```python
from build123d import *

# Parameters (mm, degrees)
F0_W      = 150
F0_H      = 98.5
F1_DEPTH  = 5
F3_W      = 70.65
F3_H      = 77.55
F3_W_2    = 68.65
F3_H_2    = 75.55
F4_DEPTH  = 1
F5_R      = 4
F5_R_2    = 2
F6_DEPTH  = 3
F7_R      = 1.5
F8_DEPTH  = 12.5
F9_R      = 2.75
F10_DEPTH = 2.5
F11_W     = 3
F11_H     = 10
F12_DEPTH = 25
F14_DEPTH = 5
F15_R     = 4
F16_DEPTH = 25
F13_W     = 1
F13_H     = 6
F17_DEPTH = 25
F18_W     = 9.35
F18_H     = 6
F19_DEPTH = 2
F20_W     = 10
F20_H     = 3
F21_DEPTH = 5
F23_DEPTH = 200


with BuildPart() as f1:
    # F0 (on Top) → F1 (new body)
    with BuildSketch(Plane.XY):
        Rectangle(F0_W, F0_H)
    extrude(amount=F1_DEPTH)

    # F3 (on face) → F4 (join)
    with BuildSketch(Plane.XY.offset(5)):
        Polygon((-66.5, -42.5), (-66.5, 42.5), (-67.5, 43.5), (-67.5, -43.5), align=None)
        Polygon((-12.5, 43.5), (-13.5, 42.5), (-13.5, -42.5), (-12.5, -43.5), align=None)
        with Locations((32.175, -0.275)):
            Rectangle(F3_W, F3_H)
        with Locations((32.175, -0.275)):
            Rectangle(F3_W_2, F3_H_2, mode=Mode.SUBTRACT)
    extrude(amount=F4_DEPTH)

    # F5 (on face) → F6 (join)
    with BuildSketch(Plane.XY.offset(5)):
        with Locations((9, 27.5)):
            Circle(F5_R)
        with Locations((9, 27.5)):
            Circle(F5_R_2, mode=Mode.SUBTRACT)
        with Locations((55.5, 27.5)):
            Circle(F5_R)
        with Locations((55.5, 27.5)):
            Circle(F5_R_2, mode=Mode.SUBTRACT)
        with Locations((55.5, -23)):
            Circle(F5_R)
        with Locations((55.5, -23)):
            Circle(F5_R_2, mode=Mode.SUBTRACT)
        with Locations((9, -23)):
            Circle(F5_R)
        with Locations((9, -23)):
            Circle(F5_R_2, mode=Mode.SUBTRACT)
    extrude(amount=F6_DEPTH)

    # F7 (on face) → F8 (cut, symmetric)
    with BuildSketch(Plane.XY.offset(5)):
        with Locations((9, 27.5)):
            Circle(F7_R)
        with Locations((55.5, 27.5)):
            Circle(F7_R)
        with Locations((9, -23)):
            Circle(F7_R)
        with Locations((55.5, -23)):
            Circle(F7_R)
        with Locations((-58, 33.5)):
            Circle(F7_R)
        with Locations((-22, 33.5)):
            Circle(F7_R)
        with Locations((-58, -33.5)):
            Circle(F7_R)
        with Locations((-22, -33.5)):
            Circle(F7_R)
        with Locations((-60, -44.25)):
            Circle(F7_R)
        with Locations((60, -44.25)):
            Circle(F7_R)
        with Locations((60, 44.25)):
            Circle(F7_R)
        with Locations((-60, 44.25)):
            Circle(F7_R)
    extrude(amount=F8_DEPTH, both=True, mode=Mode.SUBTRACT)

    # F9 (on face) → F10 (cut)
    with BuildSketch(Plane(origin=(0, 0, 0), x_dir=(1, 0, 0), z_dir=(0, 0, -1))):
        with Locations((9, 23)):
            Circle(F9_R)
        with Locations((55.5, 23)):
            Circle(F9_R)
        with Locations((9, -27.5)):
            Circle(F9_R)
        with Locations((55.5, -27.5)):
            Circle(F9_R)
        with Locations((-22, -33.5)):
            Circle(F9_R)
        with Locations((-58, -33.5)):
            Circle(F9_R)
        with Locations((-22, 33.5)):
            Circle(F9_R)
        with Locations((-58, 33.5)):
            Circle(F9_R)
        with Locations((-60, -44.25)):
            Circle(F9_R)
        with Locations((60, -44.25)):
            Circle(F9_R)
        with Locations((-60, 44.25)):
            Circle(F9_R)
        with Locations((60, 44.25)):
            Circle(F9_R)
    extrude(amount=-F10_DEPTH, mode=Mode.SUBTRACT)

    # F11 (on face) → F12 (cut)
    with BuildSketch(Plane.XY.offset(5)):
        with Locations((-71.5, 30)):
            Rectangle(F11_W, F11_H)
        with Locations((-71.5, 0)):
            Rectangle(F11_W, F11_H)
        with Locations((-71.5, -30)):
            Rectangle(F11_W, F11_H)
        with Locations((71.5, -30)):
            Rectangle(F11_W, F11_H)
        with Locations((71.5, 30)):
            Rectangle(F11_W, F11_H)
        with Locations((71.5, 0)):
            Rectangle(F11_W, F11_H)
    extrude(amount=-F12_DEPTH, mode=Mode.SUBTRACT)

    # F13 (on face) → F14 (join)
    with BuildSketch(Plane.XY.offset(5)):
        Polygon((-7.825, 29.25), (-12.5, 29.25), (-12.5, 27.25), (-11.5, 27.25), (-11.5, 21.25), (-12.5, 21.25), (-12.5, 19.25), (-7.825, 19.25), align=None)
        Polygon((-3.15, 29.25), (-7.825, 29.25), (-7.825, 19.25), (-3.15, 19.25), (-3.15, 21.25), (-4.15, 21.25), (-4.15, 27.25), (-3.15, 27.25), align=None)
    extrude(amount=F14_DEPTH)

    # F15 (on face) → F16 (cut)
    with BuildSketch(Plane.XZ.offset(-19.25)):
        with Locations((-7.825, 10)):
            Circle(F15_R)
    extrude(amount=-F16_DEPTH, mode=Mode.SUBTRACT)

    # F13 (on face) → F17 (cut)
    with BuildSketch(Plane.XY.offset(5)):
        with Locations((-12, 24.25)):
            Rectangle(F13_W, F13_H)
        with Locations((-3.65, 24.25)):
            Rectangle(F13_W, F13_H)
    extrude(amount=-F17_DEPTH, mode=Mode.SUBTRACT)

    # F18 (on face) → F19 (cut)
    with BuildSketch(Plane(origin=(0, 0, 0), x_dir=(1, 0, 0), z_dir=(0, 0, -1))):
        with Locations((-7.825, -24.25)):
            Rectangle(F18_W, F18_H)
    extrude(amount=-F19_DEPTH, mode=Mode.SUBTRACT)

    # F20 (on face) → F21 (join)
    with BuildSketch(Plane(origin=(0, 49.25, 0), x_dir=(-1, 0, 0), z_dir=(0, 1, 0))):
        with Locations((-62.5, 3.5)):
            Rectangle(F20_W, F20_H)
        with Locations((-27.5, 3.5)):
            Rectangle(F20_W, F20_H)
        with Locations((27.5, 3.5)):
            Rectangle(F20_W, F20_H)
        with Locations((62.5, 3.5)):
            Rectangle(F20_W, F20_H)
    extrude(amount=F21_DEPTH)

    # F22 (on face) → F23 (cut)
    with BuildSketch(Plane(origin=(-67.5, 0, 0), x_dir=(0, -1, 0), z_dir=(-1, 0, 0))):
        Polygon((-54.25, 5), (-54.25, 3.5), (-51.75, 5), align=None)
    extrude(amount=-F23_DEPTH, mode=Mode.SUBTRACT)


solid = f1.part
```
Check sheet for the modelled part. Datum: model origin and axes. Units: mm. A direction names the side the tool comes from. Round coordinates to 2 decimals unless told otherwise and drop trailing zeros. Loops run counter-clockwise (first coordinate to the right, second up) from the corner with the lowest first, then second, coordinate; pieces in that order, holes last. Notation, with made-up numbers: (-33.75, -25) -> (3.25, -25) arc R19 ccw to (3.25, -17) -> close; hole circle Ø3 at (64, -39). An arc over 180 degrees is marked (long way). Write item = value, one per line. Start each with the question number.
1) Gauge pin test, flat ends, axial feed: pin 1 Ø3.5 at (y, z) = (51.5, 3.5) entering from -X; pin 2 Ø1.5 at (x, y) = (-61.5, 52.5) entering from -Z; pin 3 Ø6 at (x, y) = (5, 7) entering from +Z. Record the tip position at first contact, or that the pin passes through.
2) Sectioned sample at A-A, the plane x = 44. Record the cut outline in (y, z).
3) Release check for a two-part mould opening along Y. For faces 1 (the flat face through (-62, 52, 2)), 2 (the flat face through (-7.8, 21.25, 1.6)) record: released by +Y, released by -Y, zero draft, split by the parting line, or undercut.
4) Set-up check for faces 3 (the flat face through (-73, 30, 3)), 4 (the flat face through (-32.5, 52, 3)), 5 (the flat face through (-57, 35, 2.5)), 6 (the cylindrical face through (6.05, -20.3, 6.48)): record each of +Z, -Z, +X, -X, +Y, -Y from which the full face is reachable in a straight line by a thin tool's end or side.
5) Thickness scan on probe 1 along X at (y, z) = (-7, 5.5); probe 2 along Y at (x, z) = (55.5, 3.9); probe 3 along Y at (x, z) = (9, 1.8). Record the ranges inside material, lowest first.
6) Sectioned sample at B-B, the plane y = -23. State how many separate pieces and enclosed holes the cut face has, plus the area to 4 significant figures.
Results are:
q1.pin_1 = -67.5
q1.pin_2 = 2
q1.pin_3 = 5
q2.outline = (-49.25, 0) -> (49.25, 0) -> (49.25, 5) -> (38.5, 5) -> (38.5, 6) -> (37.5, 6) -> (37.5, 5) -> (-38.05, 5) -> (-38.05, 6) -> (-39.05, 6) -> (-39.05, 5) -> (-49.25, 5) -> close
q3.face_1 = zero draft
q3.face_2 = undercut
q4.face_3 = +Z, -Z
q4.face_4 = +Z, -Z, +Y
q4.face_5 = -Z
q4.face_6 = +Z
q5.probe_1 = -67.5 to -66.5, -13.5 to -12.5, -3.15 to -2.15, 66.5 to 67.5
q5.probe_2 = -49.25 to -24.5, -21.5 to 26, 29 to 49.25
q5.probe_3 = -49.25 to -25.75, -20.25 to 24.75, 30.25 to 49.25
q6.separate_pieces = 3
q6.enclosed_holes = 0
q6.area = 735.5 mm^2
